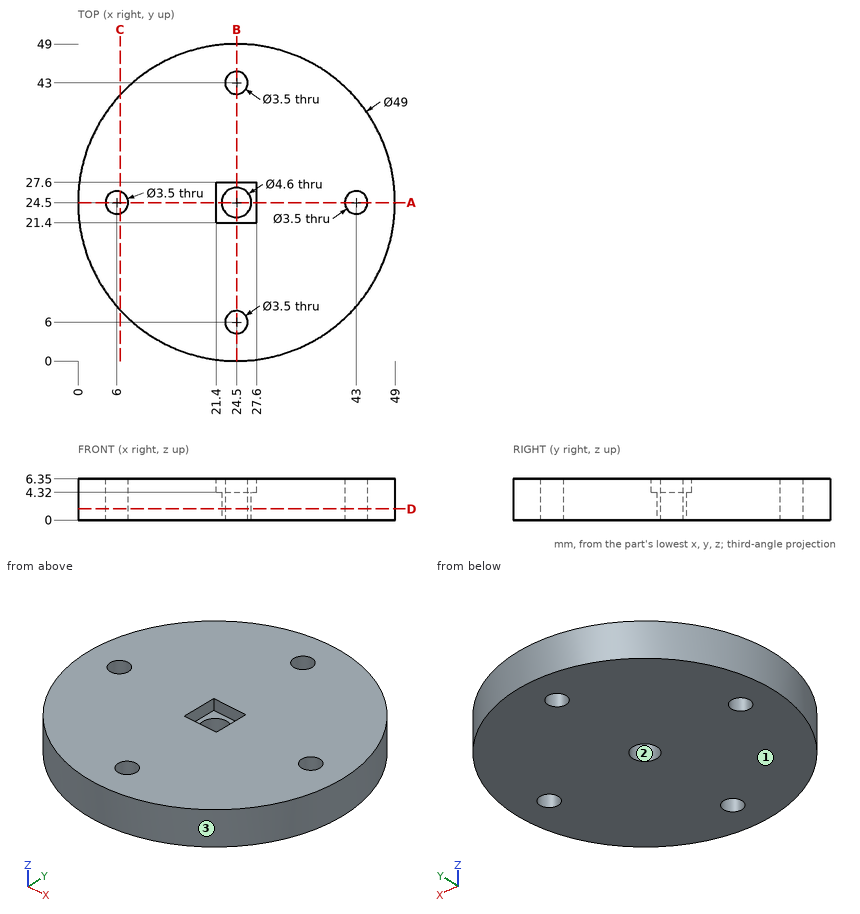
Source: three-view drawing plus pictorial views. Frame: mm from the lowest corner of the part. Give positions to 0.01 mm unless a question says otherwise; leave off trailing zeros. Order: outer loops, then holes, each group sorted by start corner. A loop starts at its lowest first (then second) coordinate and runs counter-clockwise, first axis right, second up. Notation, with made-up numbers: (14, -31.5) -> (55, -31.5) arc R6 ccw to (55, -26.5) -> close; hole circle Ø2 at (41.5, -1). An arc over 180 degrees is marked (long way). Put each result on its own line as item: value.
Q1. Material intervals for L1, parallel to Y at x = 24.5, z = 3; L2, parallel to Y at x = 22.5, z = 6.25; L3, parallel to X at y = 42, z = 3.75, sorted ascending.
Here are the results:
L1: y = 0 to 4.25, 7.75 to 22.2, 26.8 to 41.25, 44.75 to 49
L2: y = 0.08 to 21.4, 27.6 to 48.92
L3: x = 7.35 to 23.06, 25.94 to 41.65
Q2. Pin query (flat end, axial travel): pin 1 (2 mm diameter, centred on y = 23.5, z = 5.5, fed in from +X); pin 2 (1 mm diameter, centred on y = 26, z = 5, fed in from -X); pin 3 (1.6 mm diameter, centred on x = 25, z = 6, fed in from +Y); pin 4 (1 mm diameter, centred on x = 36, z = 2.5, fed in from +Y). Return the tip coordinate at first contact, or that it passes through.
Here are the results:
pin 1: stops at x = 49
pin 2: stops at x = 0.02
pin 3: stops at y = 49
pin 4: stops at y = 46.39
Q3. Section C-C, the plane x = 6.5. Return loops of the section in (y, z).
Here are the results:
outline: (7.88, 0) -> (22.82, 0) -> (22.82, 6.35) -> (7.88, 6.35) -> close; (26.18, 0) -> (41.12, 0) -> (41.12, 6.35) -> (26.18, 6.35) -> close
Q4. Section D-D, the plane z = 1.75. Return loops of the section in (x, y), then the cut area to 3 significant figures.
Here are the results:
outline: circle Ø49 at (24.5, 24.5); hole circle Ø3.5 at (6, 24.5); hole circle Ø4.6 at (24.5, 24.5); hole circle Ø3.5 at (24.5, 6); hole circle Ø3.5 at (24.5, 43); hole circle Ø3.5 at (43, 24.5)
area: 1,830 mm^2
Q5. Section A-A, the plane y = 24.5. Return loops of the section in (x, z).
Here are the results:
outline: (0, 0) -> (4.25, 0) -> (4.25, 6.35) -> (0, 6.35) -> close; (7.75, 0) -> (22.2, 0) -> (22.2, 4.32) -> (21.4, 4.32) -> (21.4, 6.35) -> (7.75, 6.35) -> close; (26.8, 0) -> (41.25, 0) -> (41.25, 6.35) -> (27.6, 6.35) -> (27.6, 4.32) -> (26.8, 4.32) -> close; (44.75, 0) -> (49, 0) -> (49, 6.35) -> (44.75, 6.35) -> close
Q6. Draft query along Y for the marked faces 1, 2 and 3. Return one class per face: released by +Y, released by -Y, zero draft, split by the parting line, or undercut.
Here are the results:
face 1: zero draft
face 2: undercut
face 3: split by the parting line
